Autodesk Inventor part; units mm, degrees
ref_plane "YZ Plane" through (0, 0, 0) normal (1, 0, 0) x (0, 1, 0)
ref_plane "XZ Plane" through (0, 0, 0) normal (0, 1, 0) x (-1, 0, 0)
ref_plane "XY Plane" through (0, 0, 0) normal (0, 0, 1) x (1, 0, 0)
sketch "Sketch1" plane through (0, 0, 0) normal (0, 1, 0) x (-1, 0, 0)
  circle A0 centre (-0.8799, 12.92) radius 2.1
  circle A1 centre (-13.5799, 0.22) radius 2.1
  circle A2 centre (-0.8799, -12.48) radius 2.1
  circle A3 centre (11.8201, 0.22) radius 2.1
  circle A4 centre (-0.8799, 0.22) radius 28.575
  line L0 (-13.5799, 0.22) -> (-0.8799, 0.22)
  circle A5 centre (-0.8799, 0.22) radius 2.54
  point P0 (0, 0)
  dimension "d0" = 57.15
  dimension "d1" = 5.08
extrude "Extrusion1" add sketch "Sketch1" along normal blind 1.5875
sketch "Sketch2" plane through (0, 0, 0) normal (0, 1, 0) x (-1, 0, 0)
  circle A0 centre (-0.8799, 0.22) radius 28.575
  circle A1 centre (-13.5799, 0.22) radius 2.1
  circle A2 centre (-0.8799, -12.48) radius 2.1
  circle A3 centre (-0.8799, 0.22) radius 2.54
  circle A4 centre (-0.8799, 12.92) radius 2.1
  circle A5 centre (11.8201, 0.22) radius 2.1
  point P0 (0, 0)
equation "\"BendRadius\" = Thickness"
equation "\"BendReliefWidth\" = Thickness"
equation "\"BendReliefDepth\" = 0.5 * Thickness"
equation "\"CornerReliefSize\" = 4 * Thickness"
equation "\"MinimumRemnant\" = 2 * Thickness"
equation "\"TransitionRadius\" = BendRadius"
equation "\"JacobiRadiusSize\" = BendRadius"
equation "\"GapSize\" = Thickness"
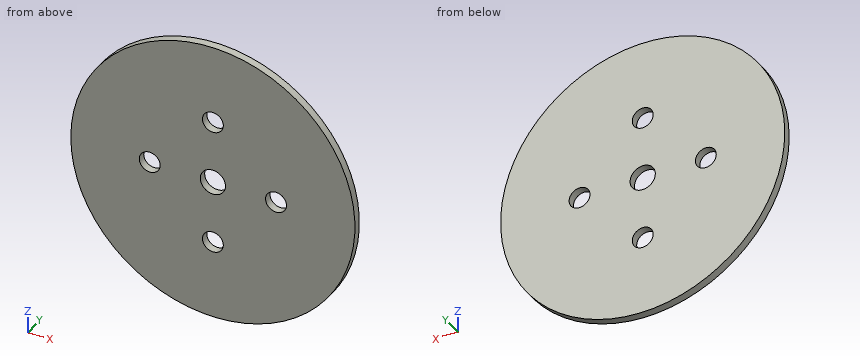
Design review of the part built by this model. Coordinates are the model's own, in mm. Give positions to 0.01 mm unless a question says otherwise; leave off trailing zeros. Loops run counter-clockwise (first coordinate to the right, second up) from the corner with the lowest first, then second, coordinate; pieces in that order, holes last. Notation, with made-up numbers: M 32,-7.75 L 54,-7.75 A26 ccw 54,18.25 Z; hole C 7.5,-33.75 d11. An arc over 180 degrees is marked long. Write item = value, one per line.
Q1. We need section C-C (z = 12.92). Give the boundary of the cut face in (x, y), plus the area to 3 significant figures.
Output values:
outline = M -24.72,0 L -1.22,0 L -1.22,1.59 L -24.72,1.59 Z; M 2.98,0 L 26.48,0 L 26.48,1.59 L 2.98,1.59 Z
area = 74.6 mm^2
Q2. To check wall thickness, follow line 1 (X direction, y = 1, z = 0); line 2 (Z direction, x = -12.5, y = 0.4); line 3 (Z direction, x = 24.5, y = 0.15). State the ranges of each line that lie inside material, in increasing order. Write a range as [from, to].
Output values:
line_1 = [-27.69, -13.91], [-9.73, -1.65], [3.41, 11.49], [15.67, 29.45]
line_2 = [-25.03, -1.77], [2.21, 25.47]
line_3 = [-15.86, 16.3]
Q3. We need section A-A (y = 0.95). Give the boundary of the cut face in (x, z) (3 decimals), plus the area to 3 significant figures.
Output values:
outline = C 0.88,0.22 d57.15; hole C -11.82,0.22 d4.2; hole C 0.88,0.22 d5.08; hole C 0.88,-12.48 d4.2; hole C 0.88,12.92 d4.2; hole C 13.58,0.22 d4.2
area = 2,490 mm^2
Q4. We need section B-B (z = 1). Give the boundary of the cut face in (x, y), plus the area to 3 significant figures.
Output values:
outline = M -27.68,0 L -13.77,0 L -13.77,1.59 L -27.68,1.59 Z; M -9.87,0 L -1.54,0 L -1.54,1.59 L -9.87,1.59 Z; M 3.3,0 L 11.63,0 L 11.63,1.59 L 3.3,1.59 Z; M 15.53,0 L 29.44,0 L 29.44,1.59 L 15.53,1.59 Z
area = 70.6 mm^2
Q5. We need section D-D (x = 21.5). Give the boundary of the cut face in (y, z), plus the area to 3 significant figures.
Output values:
outline = M 0,-19.56 L 1.59,-19.56 L 1.59,20 L 0,20 Z
area = 62.8 mm^2
Q6. Insertion check: pin 1 (2.5 mm diameter, centred on x = 0.88, z = 12.92, fed in from +Y). The pin has a flat end and moves straight along its axis. Give the tip position at first contact, or say it passes through.
Output values:
pin_1 = through
